Autodesk Inventor part; units mm, degrees
ref_plane "YZ Plane" through (0, 0, 0) normal (1, 0, 0) x (0, 1, 0)
ref_plane "XZ Plane" through (0, 0, 0) normal (0, 1, 0) x (-1, 0, 0)
ref_plane "XY Plane" through (0, 0, 0) normal (0, 0, 1) x (1, 0, 0)
sketch "Sketch1" plane through (0, 0, 0) normal (0, 0, 1) x (1, 0, 0)
  line L0 (0, 0) -> (20, 0)
  line L1 (20, 0) -> (20, 1.5)
  line L2 (20, 1.5) -> (2.35, 1.5)
  line L3 (2.35, 1.5) -> (2.15, 1.5)
  line L4 (2.15, 1.5) -> (1.67, 1.5)
  line L5 (1.65, 1.515) -> (1.65, 1.515)
  line L6 (1.65, 1.515) -> (0.415, 2.75)
  line L7 (0.415, 2.75) -> (0, 2.75)
  line L8 (0, 2.75) -> (0, 0)
  line L9 (1.65, 1.515) -> (1.65, 1.52)
  arc A0 (1.65, 1.52) -> (1.67, 1.5) centre (1.67, 1.52) ccw
  dimension "d17" = 20
  dimension "d18" = 0.415
  dimension "d19" = 1.65
  dimension "d20" = 0
  dimension "d21" = 5.5
  dimension "d22" = 3
  dimension "d23" = 3
  dimension "d25" = 45
  dimension "d26" = 0.2
  dimension "d28" = 0.02
  dimension "d29" = 17.65
  dimension "d30" = 0.02
  dimension "d52" = 0.7
revolve "Revolution1" add sketch "Sketch1" angle 360 about axis through (0, 0, 0) along (1, 0, 0)
thread "Thread1"
sketch "Sketch2" plane through (0, 0, 0) normal (-1, 0, 0) x (0, 0, 1)
  circle A0 centre (0, 0) radius 1.4 construction
  circle A1 centre (0, 0) radius 0.98 construction
  line L0 (0, 0) -> (0.8487, 0.49)
  line L1 (0, 0) -> (0.98, 0) construction
  line L2 (0, 0) -> (0.8487, -0.49)
  line L3 (0, 0) -> (0.98, 0) construction
  line L4 (0.8487, 0.49) -> (1.4, 0)
  line L5 (1.4, 0) -> (0.8487, -0.49)
  dimension "d34" = 2.8
  dimension "d35" = 1.96
  dimension "d39" = 30
  dimension "d40" = 330
extrude "Extrusion1" cut sketch "Sketch2" against normal blind 0.83
pattern_circular "Circular Pattern1" count 6 over 360 about axis through (-10, 0, 0) along (1, 0, 0) of "Extrusion1"
fillet "Fillet1" radius 0.3 12 edges at (0.415, 0.49, 0.8487) (0.415, 0, 1.4) (0.415, -0.49, 0.8487) (0.415, -0.98, 0) (0.415, -1.2124, 0.7) (0.415, -1.2124, -0.7) (0.415, -0.49, -0.8487) (0.415, 0, -1.4) (0.415, 0.49, -0.8487) (0.415, 1.2124, -0.7) (0.415, 0.98, 0) (0.415, 1.2124, 0.7)
equation "\"d32\" = b"
equation "\"d34\" = A_"
equation "\"d35\" = 0.7 * A_"
equation "\"d43\" = t"
equation "\"d48\" = v"
equation "\"d17\" = l_"
equation "\"d18\" = 0.5 * t"
equation "\"d19\" = k"
equation "\"d21\" = dk"
equation "\"d22\" = d"
equation "\"d23\" = ds_"
equation "\"d25\" = 0.5 * headAngle"
equation "\"d26\" = x"
equation "\"d28\" = r"
equation "\"d29\" = b"
properties part number "Šroub se zápustnou hlavou a šestiramennou drážkou ISO 14581 - M3x20-4.8" material "Ocel, měkká"
Work out the finished part from the listing and answer in its coordinate system (mm). Give positions to 0.01 mm unless a question says otherwise; leave off trailing zeros. Order: outer loops, then holes, each group sorted by start corner. A loop starts at its lowest first (then second) coordinate and runs counter-clockwise, first axis right, second up. Notation, with made-up numbers: (74, 64.5) - (101, 64.5) arc R15 ccw to (101, 80.5) - close; hole circle Ø11 at (-13.75, 61). An arc over 180 degrees is marked (long way). One line per item, written item: value. Start each with the question number.
1. For a pull along Y with two mould halves and no side action, classify faces 1 (the face through (10.71, -1.5, -0.07)), 2 (the face through (0.83, 0, 0)), 3 (the face through (0, 1.2, 0)) as released by +Y, released by -Y, zero draft, split by the parting line, or undercut.
2. Consider line 1 (X direction, y = -1.35, z = 2.2); line 2 (Y direction, x = 2.5, z = -0.1); line 3 (X direction, y = 0.85, z = -0.65). Determine where each line is inside the solid, lowest interval first.
3. Section A-A, the plane y = 0 is taken. Write down the section's boundary in (x, z) (3 decimals).
4. Section B-B, the plane x = 12 is taken. Write down the section's boundary in (y, z), then the cut area to 3 significant figures.
5. Each of these flat-tipped pins is pushed along its axis until it touches: pin 1 Ø1 at (x, y) = (13.5, -0.5) entering from +Z; pin 2 Ø1.5 at (x, z) = (5, 0.5) entering from -Y. Where does it stop, or does it pass through?
Filled sheet:
1. face 1: split by the parting line
1. face 2: undercut
1. face 3: zero draft
2. line 1: 0 to 0.58
2. line 2: -1.5 to 1.5
2. line 3: 0.83 to 20
3. outline: (0, -2.75) - (0.415, -2.75) - (1.65, -1.515) arc R0.02 cw to (1.67, -1.5) - (20, -1.5) - (20, 1.5) - (1.67, 1.5) arc R0.02 cw to (1.651, 1.515) - (0.415, 2.75) - (0, 2.75) - (0, 1.248) - (0.83, 1.248) - (0.83, -1.248) - (0, -1.248) - close
4. outline: circle Ø3 at (0, 0)
4. area: 7.07 mm²
5. pin 1: z = 1.5
5. pin 2: y = -1.5
